from build123d import *

# Parameters (mm, degrees)
F0_W     = 50.8
F0_H     = 96.52
F0_W_2   = 25.4
F0_H_2   = 25.4
F1_DEPTH = 25.4
F2_R     = 5.08


with BuildPart() as f1:
    # F0 (on Top) → F1 (new body)
    with BuildSketch(Plane.XY):
        Rectangle(F0_W, F0_H)
        with BuildLine():
            Line((25.4, -48.26), (-25.4, -48.26))
            add(Edge.make_bspline(
                [(-25.4, -48.26), (-25.400003, -73.229496), (-9.901697, -74.52103), (25.4, -73.66)],
                knots=[0, 0, 0, 0, 56.796127, 56.796127, 56.796127, 56.796127], degree=3))
            Line((25.4, -73.66), (25.4, -48.26))
        make_face()
        with Locations((38.1, -60.96)):
            Rectangle(F0_W_2, F0_H_2)
    extrude(amount=F1_DEPTH)

    # F2
    f2_edges = [f1.edges().sort_by_distance(p)[0] for p in [
        (25.4, 0, 25.4),
        (38.1, -48.26, 25.4),
        (38.1, -48.26, 0),
        (25.4, 0, 0),
        (25.4, -48.26, 12.7),
    ]]
    fillet(f2_edges, radius=F2_R)

    # F3: F1 across face


with BuildPart() as f1_1:
    add(f1.part)
    add(f1.part.mirror(Plane(origin=(50.8, -61.162023, 12.7), x_dir=(0, 1, 0), z_dir=(1, 0, 0))))


solid = f1_1.part
Verification items for the finished model (mm, model axes). A direction names the side the tool comes from. Give positions to 0.01 mm unless a question says otherwise; leave off trailing zeros. Order: outer loops, then holes, each group sorted by start corner. A loop starts at its lowest first (then second) coordinate and runs counter-clockwise, first axis right, second up. Notation, with made-up numbers: M -26.5,-3.5 L -13.5,-3.5 A8 cw -13.5,7.5 Z; hole C 14.25,47.25 d7. An arc over 180 degrees is marked long. Answer as a JSON object with one key per item and string values. Group by question number.
1) Access from +Z, -Z, +X, -X, +Y, -Y to the whole of each face (thin tool, end or side, straight path). Record for faces 4 (the face through (23.951, 3.18, 1.528)), 5 (the face through (74.672, -46.811, 12.807)), 6 (the face through (51, -73.66, 13)), 7 (the face through (50.516, -49.709, 23.872)).
2) Depth check by flat-ended pin: pin 1 Ø1.5 at (x, z) = (34, 20) entering from -Y; pin 2 Ø1 at (x, y) = (22.5, -45) entering from +Z; pin 3 Ø1.5 at (x, z) = (-4, 18) entering from -Y. Enter the tip coordinate at first touch or a pass-through.
3) Cross-section at A-A (y = -21.5). Enter the section's corners in (x, z), then the cut area to 3 significant figures.
4) Mould release check, pull along X, two halves, no side actions. Record for faces 1 (the face through (76.2, 2, 13)), 2 (the face through (127, -1, 13)), 3 (the face through (0, 48.26, 13)): released by +X, released by -X, zero draft, split by the parting line, or undercut.
5) Scan lines: line 1 along X through (y, z) = (-11, 10); line 2 along Y through (x, z) = (52, 5); line 3 along X through (y, z) = (2.5, 23). Record each from-to range of solid material in increasing order. Write a range as [from, to].
6) Cross-section at B-B (x = 40). Enter the section's corners in (y, z), then the cut area to 3 significant figures.
Result sheet:
{
 "1": {"face 4": "-Z, +Y", "face 5": "+Z, -Z, +Y", "face 6": "+Z, -Z, -Y", "face 7": "+Z, +Y"},
 "2": {"pin 1": "stops at y = -73.66", "pin 2": "stops at z = 25.18", "pin 3": "stops at y = -73.03"},
 "3": {"outline": "M -25.4,0 L 20.32,0 A5.08 ccw 25.4,5.08 L 25.4,20.32 A5.08 ccw 20.32,25.4 L -25.4,25.4 Z; M 76.2,5.08 A5.08 ccw 81.28,0 L 127,0 L 127,25.4 L 81.28,25.4 A5.08 ccw 76.2,20.32 Z", "area": "2,560 mm2"},
 "4": {"face 1": "undercut", "face 2": "released by +X", "face 3": "zero draft"},
 "5": {"line 1": "x = [-25.4, 25.4], [76.2, 127]", "line 2": "y = [-73.66, -48.26]", "line 3": "x = [-25.4, 24.64], [76.96, 127]"},
 "6": {"outline": "M -73.66,0 L -53.34,0 A5.08 ccw -48.26,5.08 L -48.26,20.32 A5.08 ccw -53.34,25.4 L -73.66,25.4 Z", "area": "634 mm2"}
}
